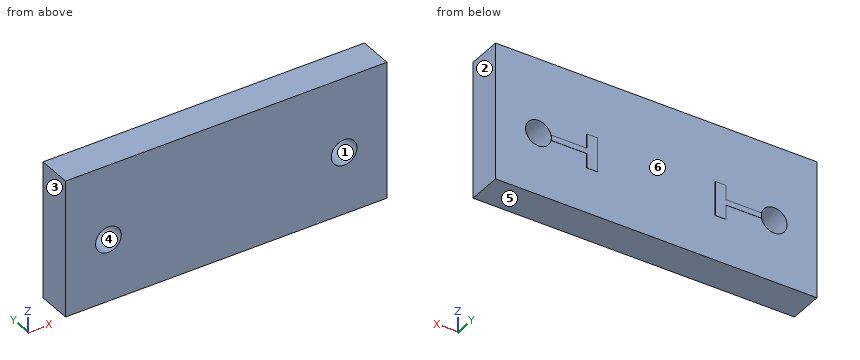
```python
from build123d import *

# Parameters (mm, degrees)
SKETCH1_W           = 15
SKETCH1_H           = 4
BOSS_EXTRUDE1_DEPTH = 1.6
SKETCH3_R           = 0.6
CUT_EXTRUDE1_DEPTH  = 1.6
SKETCH2_W           = 0.5
SKETCH2_H           = 1.6
BOSS_EXTRUDE2_DEPTH = 0.01
BOSS_EXTRUDE3_DEPTH = 0.01
SKETCH5_W           = 15
SKETCH5_H           = 1.6
BOSS_EXTRUDE4_DEPTH = 1.5
SKETCH6_W           = 15
SKETCH6_H           = 1.6
BOSS_EXTRUDE5_DEPTH = 0.9


with BuildPart() as part:
    # Sketch1 → Boss-Extrude1 (new body)
    with BuildSketch(Plane(origin=(0, 0, 0), x_dir=(1, 0, 0), z_dir=(0, 1, 0))):
        Rectangle(SKETCH1_W, SKETCH1_H)
    extrude(amount=BOSS_EXTRUDE1_DEPTH)

    # Sketch3 → Cut-Extrude1 (cut)
    with BuildSketch(Plane(origin=(0, 1.6, 0), x_dir=(1, 0, 0), z_dir=(0, 1, 0))):
        with Locations((5.5, 0)):
            Circle(SKETCH3_R)
        with Locations((-5.5, 0)):
            Circle(SKETCH3_R)
    extrude(amount=-CUT_EXTRUDE1_DEPTH, mode=Mode.SUBTRACT)

    # Sketch2 → Boss-Extrude2 (add)
    with BuildSketch(Plane(origin=(0, 1.6, 0), x_dir=(1, 0, 0), z_dir=(0, 1, 0))):
        with Locations((-3, 0)):
            Rectangle(SKETCH2_W, SKETCH2_H)
        with Locations((3, 0)):
            Rectangle(SKETCH2_W, SKETCH2_H)
    extrude(amount=BOSS_EXTRUDE2_DEPTH)

    # Sketch4 → Boss-Extrude3 (add)
    with BuildSketch(Plane(origin=(0, 1.6, 0), x_dir=(1, 0, 0), z_dir=(0, 1, 0))):
        with BuildLine():
            Line((3.25, -0.125), (4.913165, -0.125))
            ThreePointArc((4.913165, -0.125), (4.9, 0), (4.913165, 0.125))
            Line((4.913165, 0.125), (3.25, 0.125))
            Line((3.25, 0.125), (3.25, -0.125))
        make_face()
        with BuildLine():
            Line((-3.25, 0.125), (-4.913165, 0.125))
            ThreePointArc((-4.913165, 0.125), (-4.9033, 0.062846), (-4.9, 0))
            ThreePointArc((-4.9, 0), (-4.9033, -0.062846), (-4.913165, -0.125))
            Line((-4.913165, -0.125), (-3.25, -0.125))
            Line((-3.25, -0.125), (-3.25, 0.125))
        make_face()
    extrude(amount=BOSS_EXTRUDE3_DEPTH)

    # Sketch5 → Boss-Extrude4 (add)
    with BuildSketch(Plane.XY.offset(2)):
        with Locations((0, 0.8)):
            Rectangle(SKETCH5_W, SKETCH5_H)
    extrude(amount=BOSS_EXTRUDE4_DEPTH)

    # Sketch6 → Boss-Extrude5 (add)
    with BuildSketch(Plane(origin=(0, 0, -2), x_dir=(-1, 0, 0), z_dir=(0, 0, -1))):
        with Locations((0, 0.8)):
            Rectangle(SKETCH6_W, SKETCH6_H)
    extrude(amount=BOSS_EXTRUDE5_DEPTH)


solid = part.part
```
Source: CAD feature listing. Evaluate the final solid. Frame: model axes, mm. Face numbers are marked on the shaded views. A direction names the side the tool comes from. Coordinates: 2 decimals unless noted, no trailing zeros. Order: outer loops, then holes, each group sorted by start corner. A loop starts at its lowest first (then second) coordinate and runs counter-clockwise, first axis right, second up. Notation, with made-up numbers: M 9.25,-30.75 L 66.25,-30.75 A37 ccw 66.25,6.25 Z; hole C 63.5,84.25 d9. An arc over 180 degrees is marked long. Write each question's results on one line, items separated by ' | '. Start each with the question number.
1) Line query: line 1 (X direction, y = 0.75, z = 0); line 2 (X direction, y = 0.1, z = 0.25); line 3 (Y direction, x = 6.25, z = 1.5). Output: solid intervals per line, ascending. Write a range as from..to.
2) Access query for the marked faces 5 and 6. Directions: +Z, -Z, +X, -X, +Y, -Y. A direction counts if a zero-diameter tool reaches every point of the face in a straight line with its end or side. Return the directions, or none.
3) Section query B-B (y = 1.1). Return the cut outline in (x, z).
4) Section query A-A (x = -5.5). Return the cut outline in (y, z), plus the area to 3 significant figures.
5) Draft query along X for the marked faces 1, 2, 3 and 4. Return one class per face: released by +X, released by -X, zero draft, split by the parting line, or undercut.
Answers:
1) line 1: x = -7.5..-6.1, -4.9..4.9, 6.1..7.5 | line 2: x = -7.5..-6.05, -4.95..4.95, 6.05..7.5 | line 3: y = 0..1.6
2) face 5: -Z, +X, -X, +Y, -Y | face 6: +Y
3) outline: M -7.5,-2.9 L 7.5,-2.9 L 7.5,3.5 L -7.5,3.5 Z; hole C -5.5,0 d1.2; hole C 5.5,0 d1.2
4) outline: M 0,-2.9 L 1.6,-2.9 L 1.6,-0.6 L 0,-0.6 Z; M 0,0.6 L 1.6,0.6 L 1.6,3.5 L 0,3.5 Z | area: 8.32 mm^2
5) face 1: undercut | face 2: released by +X | face 3: released by -X | face 4: undercut
